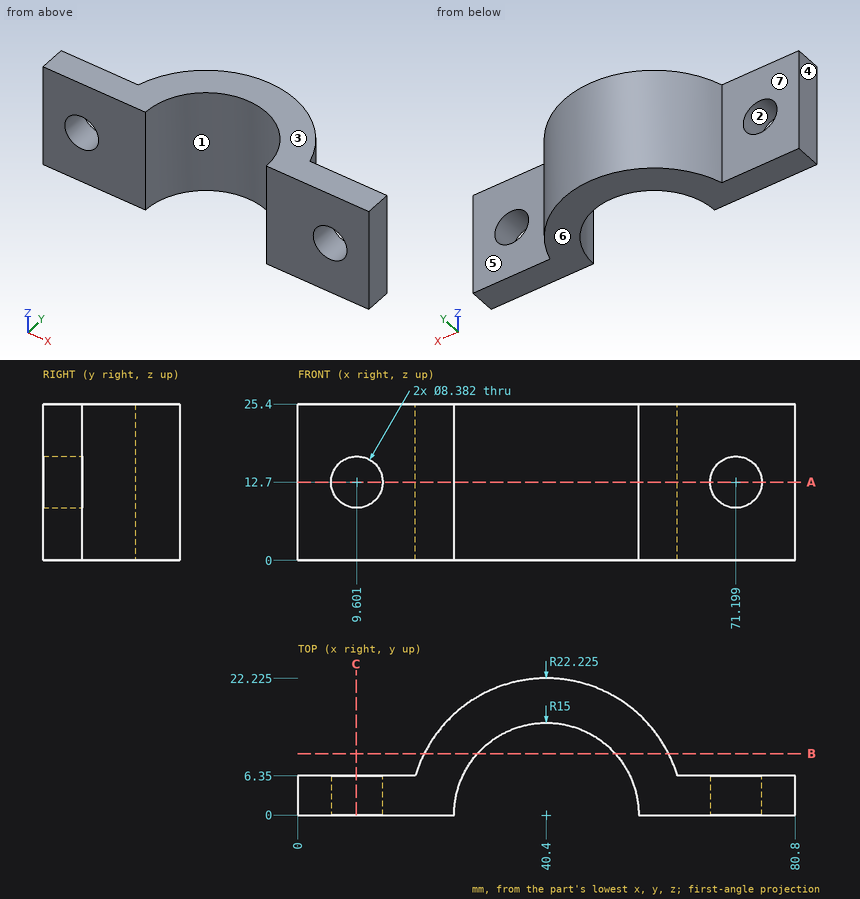
Answer from the drawing. Dimensions are ordinates in mm from the lowest x, y and z of the part. A direction names the side the tool comes from. Coordinates: 2 decimals unless noted, no trailing zeros. Order: outer loops, then holes, each group sorted by start corner. A loop starts at its lowest first (then second) coordinate and runs counter-clockwise, first axis right, second up. Notation, with made-up numbers: (33.25, -15.5) - (87.25, -15.5) arc R10 ccw to (87.25, 2.5) - close; hole circle Ø10 at (-30, 36.25). An arc over 180 degrees is marked (long way). Put each result on its own line as item: value. Start each with the question number.
1) Find section C-C (x = 9.5). Give the vertices of the cut face in (y, z).
2) For a pull along X with two mould halves and no side action, classify the marked faces 1, 2, 3 and 4 as released by +X, released by -X, zero draft, split by the parting line, or undercut.
3) Find the intervals of material crossed by line 1 (Y direction, x = 64, z = 21.75); line 2 (Z direction, x = 73, y = 1) (1 decimal); line 3 (X direction, y = 13, z = 17) (1 decimal), in increasing order. Write a range as from..to.
4) Find section B-B (y = 10). Give the vertices of the cut face in (x, z), plus the area to 3 significant figures.
5) Flat-ended cylindrical pins translate along their axes: pin 1 (5 mm diameter, centred on x = 9.6, z = 12.7, fed in from -Y); pin 2 (5.5 mm diameter, centred on x = 6, z = 11, fed in from +Y); pin 3 (4 mm diameter, centred on y = 9, z = 12, fed in from -X); pin 4 (2 mm diameter, centred on x = 46, z = 20.5, fed in from +Y). Find the tip coordinate at first contact, or state that the pin passes through.
6) For the marked faces 5, 6 and 7, determine the directions among +Z, -Z, +X, -X, +Y, -Y from which every point of the face is accessible in a straight line to the end or side of a thin tool.
7) Find section A-A (z = 12.7). State how many separate pieces and enclosed holes the cut face has, plus the area to 3 significant figures.
Results list:
1. outline: (0, 0) - (6.35, 0) - (6.35, 8.51) - (0, 8.51) - close; (0, 16.89) - (6.35, 16.89) - (6.35, 25.4) - (0, 25.4) - close
2. face 1: undercut
2. face 2: undercut
2. face 3: zero draft
2. face 4: released by -X
3. line 1: y = 0..6.35
3. line 2: z = 0..8.9, 16.5..25.4
3. line 3: x = 22.4..32.9, 47.9..58.4
4. outline: (20.55, 0) - (29.22, 0) - (29.22, 25.4) - (20.55, 25.4) - close; (51.58, 0) - (60.25, 0) - (60.25, 25.4) - (51.58, 25.4) - close
4. area: 440 mm^2
5. pin 1: passes through
5. pin 2: stops at y = 6.35
5. pin 3: stops at x = 19.31
5. pin 4: stops at y = 21.74
6. face 5: +Z, -Z, +X, +Y
6. face 6: -Z, +X, -X, +Y, -Y
6. face 7: +Z, -Z, -X, +Y
7. separate pieces: 3
7. enclosed holes: 0
7. area: 551 mm^2
